```python
from build123d import *

# Parameters (mm, degrees)
SKETCH1_R           = 4.25
BOSS_EXTRUDE1_DEPTH = 54.11518367
CUT_EXTRUDE1_DEPTH  = 6.6
CHAMFER1_SIZE       = 0.5
CUT_EXTRUDE2_DEPTH  = 6.6
CHAMFER2_SIZE       = 0.5


with BuildPart() as part:
    # Sketch1 → Boss-Extrude1 (new body)
    with BuildSketch(Plane(origin=(0, 0, 0), x_dir=(1, 0, 0), z_dir=(0, 1, 0))):
        Circle(SKETCH1_R)
    extrude(amount=BOSS_EXTRUDE1_DEPTH)

    # Sketch2 → Cut-Extrude1 (cut)
    with BuildSketch(Plane(origin=(0, 54.11518367, 0), x_dir=(1, 0, 0), z_dir=(0, 1, 0))):
        Polygon((0, -2.79), (0, 2.79), (-1.610807251, 2.79), (-3.221614502, 0), (-1.610807251, -2.79), align=None)
        Polygon((1.610807251, 2.79), (0, 2.79), (0, -2.79), (1.610807251, -2.79), (3.221614502, 0), align=None)
    extrude(amount=-CUT_EXTRUDE1_DEPTH, mode=Mode.SUBTRACT)

    # Chamfer1
    chamfer1_edges = [part.edges().sort_by_distance(p)[0] for p in [
        (-2.416210877, 54.11518367, 1.395),
        (0, 54.11518367, 2.79),
        (2.416210877, 54.11518367, 1.395),
        (2.416210877, 54.11518367, -1.395),
        (0, 54.11518367, -2.79),
        (-2.416210877, 54.11518367, -1.395),
    ]]
    chamfer(chamfer1_edges, length=CHAMFER1_SIZE)

    # Sketch3 → Cut-Extrude2 (cut)
    with BuildSketch(Plane.XZ):
        Polygon((-1.361513121, 2.91977431), (1.361513121, -2.91977431), (-1.847842165, -2.638992105), (-3.209355286, 0.280782205), align=None)
        Polygon((1.847842165, 2.638992105), (-1.361513121, 2.91977431), (1.361513121, -2.91977431), (3.209355286, -0.280782205), align=None)
    extrude(amount=-CUT_EXTRUDE2_DEPTH, mode=Mode.SUBTRACT)

    # Chamfer2
    chamfer2_edges = [part.edges().sort_by_distance(p)[0] for p in [
        (-0.243164522, 0, -2.779383208),
        (2.285434204, 0, -1.600278257),
        (2.528598726, 0, 1.17910495),
        (0.243164522, 0, 2.779383208),
        (-2.285434204, 0, 1.600278257),
        (-2.528598726, 0, -1.17910495),
    ]]
    chamfer(chamfer2_edges, length=CHAMFER2_SIZE)


solid = part.part
```
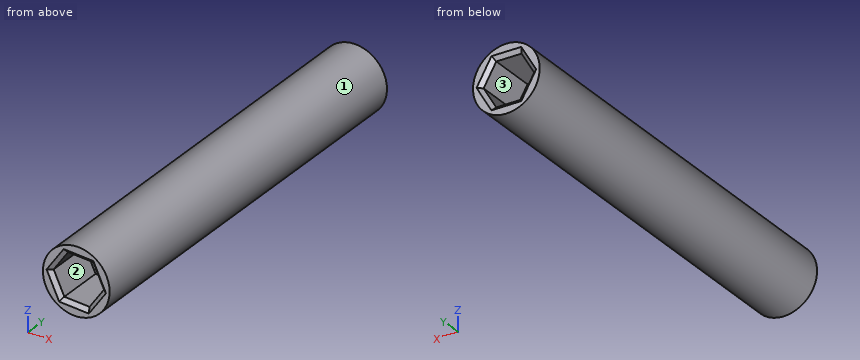
Geometry check sheet. Reference: the model listing, model coordinates, mm. Face numbers are marked on the shaded views. A direction names the side the tool comes from. Give positions to 0.01 mm unless a question says otherwise; leave off trailing zeros. Write each loop counter-clockwise with the first axis right and the second up, starting at its lowest first coordinate (ties: lowest second). Pieces come first, ordered by that corner, then holes.
1) Section check A-A, the plane y = 49. Record the boundary of the cut face in (x, z), and give its area (3 significant figures).
2) Section check C-C, the plane x = 0.25. Record the boundary of the cut face in (y, z), and give its area (3 significant figures).
3) Gauge pin test, flat ends, axial feed: pin 1 (1.7 mm diameter, centred on x = 0.5, z = 1, fed in from +Y); pin 2 (1 mm diameter, centred on y = 43, z = -2.5, fed in from -X); pin 3 (1.8 mm diameter, centred on x = 1.5, z = -0.5, fed in from -Y). Record the tip position at first contact, or that the pin passes through.
4) Section check B-B, the plane z = -1.5. Record the boundary of the cut face in (x, y).
5) Access from +Z, -Z, +X, -X, +Y, -Y to the whole of each face (thin tool, end or side, straight path). Record for the marked faces 1, 2 and 3.
6) Material ranges on L1, parallel to X at y = 36.5, z = -0.25; L2, parallel to X at y = 46.5, z = -2.5; L3, parallel to Y at x = 3.5, z = 0.5, recorded low to high.
Computed:
1. outline: circle Ø8.5 at (0, 0); hole (-3.22, 0) - (-1.61, -2.79) - (1.61, -2.79) - (3.22, 0) - (1.61, 2.79) - (-1.61, 2.79) - close
1. area: 29.8 mm2
2. outline: (0, -4.24) - (54.12, -4.24) - (54.12, -3.29) - (53.62, -2.79) - (47.52, -2.79) - (47.52, 2.79) - (53.62, 2.79) - (54.12, 3.29) - (54.12, 4.24) - (0, 4.24) - (0, 3.28) - (0.5, 2.78) - (6.6, 2.78) - (6.6, -2.82) - (0.5, -2.82) - (0, -3.32) - close
2. area: 385 mm2
3. pin 1: stops at y = 47.52
3. pin 2: stops at x = -3.75
3. pin 3: stops at y = 6.6
4. outline: (-3.98, 0) - (-2.93, 0) - (-2.38, 0.5) - (-2.38, 6.6) - (2.36, 6.6) - (2.36, 0.5) - (2.97, 0) - (3.98, 0) - (3.98, 54.12) - (2.93, 54.12) - (2.36, 53.62) - (2.36, 47.52) - (-2.36, 47.52) - (-2.36, 53.62) - (-2.93, 54.12) - (-3.98, 54.12) - close
5. face 1: +Y, -Y
5. face 2: -Y
5. face 3: +Y
6. L1: x = -4.24 to 4.24
6. L2: x = -3.44 to 3.44
6. L3: y = 0 to 54.11
